Autodesk Inventor part; units mm, degrees
ref_plane "YZ Plane" through (0, 0, 0) normal (1, 0, 0) x (0, 1, 0)
ref_plane "XZ Plane" through (0, 0, 0) normal (0, 1, 0) x (-1, 0, 0)
ref_plane "XY Plane" through (0, 0, 0) normal (0, 0, 1) x (1, 0, 0)
sketch "Skizze1" plane through (0, 0, 0) normal (0, 1, 0) x (-1, 0, 0)
  line L0 (0, 0) -> (188, 0)
  line L1 (188, 0) -> (188, -400)
  line L2 (188, -400) -> (0, -400)
  line L3 (0, -400) -> (0, 0)
  dimension "d1" = 188
  dimension "d2" = 400
extrude "Extrusion1" add sketch "Skizze1" along normal blind 15
sketch "Skizze2" plane through (0, 15, 0) normal (0, 1, 0) x (1, 0, 0)
  line L0 (-173, 15) -> (-155, 15)
  line L1 (-155, 15) -> (-155, 385)
  line L2 (-155, 385) -> (-173, 385)
  line L3 (-173, 385) -> (-173, 15)
  line L4 (-43, 15) -> (-61, 15)
  line L5 (-61, 15) -> (-61, 150)
  line L6 (-61, 150) -> (-43, 150)
  line L7 (-43, 150) -> (-43, 15)
  line L8 (-43, 385) -> (-61, 385)
  line L9 (-61, 385) -> (-61, 250)
  line L10 (-61, 250) -> (-43, 250)
  line L11 (-43, 250) -> (-43, 385)
  line L12 (-188, 0) -> (0, 0)
  line L13 (0, 0) -> (0, 400)
  dimension "d5" = 18
  dimension "d6" = 370
  dimension "d7" = 18
  dimension "d8" = 135
  dimension "d9" = 135
  dimension "d10" = 18
  dimension "d11" = 15
  dimension "d12" = 150
  dimension "d13" = 250
  dimension "d14" = 43
  dimension "d15" = 155
  dimension "d16" = 43
extrude "Extrusion2" add sketch "Skizze2" along normal blind 15
sketch "Skizze3" plane through (0, 30, 0) normal (0, 1, 0) x (1, 0, 0)
  point P0 (0, 0)
  point P1 (-52, 45)
  point P2 (-52, 120)
  point P3 (-52, 280)
  point P4 (-52, 355)
  point P5 (-164, 355)
  point P6 (-164, 200)
  point P7 (-164, 45)
hole "Bohrung1" at (-52, 30, -45) at (-52, 30, -120) at (-52, 30, -280) at (-52, 30, -355) at (-164, 30, -355) at (-164, 30, -200) at (-164, 30, -45) direction (0, -1, 0) diameter 4.5 depth 25 tip angle 118 countersink diameter 9 countersink angle 90
sketch "Skizze4" plane through (0, 0, 0) normal (0, -1, 0) x (1, 0, 0)
  line L0 (0, 0) -> (-188, 0)
  line L1 (0, -400) -> (0, 0)
  point P0 (-23, -200)
  point P1 (-23, -100)
  point P2 (-23, -300)
  dimension "d26" = 100
  dimension "d27" = 200
  dimension "d28" = 300
  dimension "d29" = 23
  dimension "d30" = 23
  dimension "d31" = 23
hole "Bohrung2" at (-23, 0, -100) at (-23, 0, -200) at (-23, 0, -300) direction (0, 1, 0) diameter 6.5 end through all countersink diameter 11.3 countersink angle 90
properties part number "frontHolz" material "Pappel"
Geometry: final body of the model. Coordinates: model frame, mm. A direction names the side the tool comes from. Coordinates: 2 decimals unless noted, no trailing zeros. Order: outer loops, then holes, each group sorted by start corner. A loop starts at its lowest first (then second) coordinate and runs counter-clockwise, first axis right, second up. Notation, with made-up numbers: (66.5, 81.25) - (88.5, 81.25) arc R21 ccw to (88.5, 116.25) - close; hole circle Ø8 at (8, 34). An arc over 180 degrees is marked (long way). Use one line per item in the form item = value.
1) Section C-C (x = -121.5). Return loops of the section in (y, z).
Solutions:
outline = (0, -400) - (15, -400) - (15, 0) - (0, 0) - close
2) Ray query, L1, parallel to Z at x = -23, y = 8.5; L2, parallel to Z at x = -52, y = 19.5; L3, parallel to X at y = 12.75, z = -120. Return the intervals inside material, ascending.
Solutions:
L1 = -400 to -303.25, -296.75 to -203.25, -196.75 to -103.25, -96.75 to 0
L2 = -385 to -357.25, -352.75 to -282.25, -277.75 to -250, -150 to -122.25, -117.75 to -47.25, -42.75 to -15
L3 = -188 to -54.25, -49.75 to 0
3) Pin query (flat end, axial travel): pin 1 (5 mm diameter, centred on x = -23, z = -100, fed in from -Y); pin 2 (6 mm diameter, centred on y = 11.5, z = -138.5, fed in from +X); pin 3 (7.5 mm diameter, centred on y = 25, z = -97, fed in from +X); pin 4 (16.5 mm diameter, centred on x = -48.5, y = 24.5, fed in from +Z). Return the tip coordinate at first contact, or that it passes through.
Solutions:
pin_1 = through
pin_2 = 0
pin_3 = -43
pin_4 = -15
4) Section B-B (z = -185). Return loops of the section in (x, y), then the cut area to 3 significant figures.
Solutions:
outline = (-188, 0) - (0, 0) - (0, 15) - (-155, 15) - (-155, 30) - (-173, 30) - (-173, 15) - (-188, 15) - close
area = 3,090 mm^2
5) Set-up query: faces 1 (the face through (-155, 22, -197)), 2 (the face through (-52, 22, -15)), 3 (the face through (-188, 7, -197)), 4 (the face through (-52, 30, -83)), 5 (the face through (-52, 22, -250)). Return all of +Z, -Z, +X, -X, +Y, -Y with unobstructed straight access to the full face (end or side cutting, diameter ignored); none if empty.
Solutions:
face_1 = +Z, -Z, +Y
face_2 = +Z, +X, -X, +Y
face_3 = +Z, -Z, -X, +Y, -Y
face_4 = +Z, -Z, +X, -X, +Y
face_5 = +X, +Y
6) Mould query, pull axis Z, two halves, no side actions, for faces 6 (the face through (-93, 7, 0)), 7 (the face through (-43, 22, -317)), 8 (the face through (-164, 22, -385)), 9 (the face through (-51.28, 27.89, -277.72)). Classes: +Z half, -Z half, draft (parallel to the pull), parting line (faces both ways), or undercut.
Solutions:
face_6 = +Z half
face_7 = draft
face_8 = -Z half
face_9 = undercut
7) Section A-A (y = 23.5). State how many separate pieces and enclosed holes the cut face has, then the cut area to 3 significant figures.
Solutions:
separate_pieces = 3
enclosed_holes = 7
area = 11,400 mm^2
